Design review of the part built by this model. Coordinates are the model's own, in mm. Give positions to 0.01 mm unless a question says otherwise; leave off trailing zeros. Loops run counter-clockwise (first coordinate to the right, second up) from the corner with the lowest first, then second, coordinate; pieces in that order, holes last. Notation, with made-up numbers: (24, 28.5) - (66, 28.5) arc R14 cw to (66, 45.5) - close; hole circle Ø1 at (85.25, 58). An arc over 180 degrees is marked (long way). One line per item, written item: value. Start each with the question number.
```python
from build123d import *

# Parameters (mm, degrees)
SKETCH1_R           = 37.5
SKETCH1_R_2         = 26
SKETCH1_R_3         = 1
SKETCH1_R_4         = 1.5
BOSS_EXTRUDE1_DEPTH = 7


with BuildPart() as part:
    # Sketch1 → Boss-Extrude1 (new body)
    with BuildSketch(Plane(origin=(0, 0, 0), x_dir=(1, 0, 0), z_dir=(0, 1, 0))):
        with Locations(Location((0, 0, 0), (0, 0, 270))):
            Circle(SKETCH1_R)
        with Locations(Location((0, 0, 0), (0, 0, 270))):
            Circle(SKETCH1_R_2, mode=Mode.SUBTRACT)
        with Locations(Location((0, 30, 0), (0, 0, 270))):
            Circle(SKETCH1_R_3, mode=Mode.SUBTRACT)
        with Locations(Location((25.980762114, 15, 0), (0, 0, 270))):
            Circle(SKETCH1_R_3, mode=Mode.SUBTRACT)
        with Locations(Location((25.980762114, -15, 0), (0, 0, 270))):
            Circle(SKETCH1_R_3, mode=Mode.SUBTRACT)
        with Locations(Location((0, -30, 0), (0, 0, 270))):
            Circle(SKETCH1_R_3, mode=Mode.SUBTRACT)
        with Locations(Location((-25.980762114, -15, 0), (0, 0, 270))):
            Circle(SKETCH1_R_3, mode=Mode.SUBTRACT)
        with Locations(Location((-25.980762114, 15, 0), (0, 0, 270))):
            Circle(SKETCH1_R_3, mode=Mode.SUBTRACT)
        with Locations(Location((-33.80740392, -9.058666579, 0), (0, 0, 270))):
            Circle(SKETCH1_R_4, mode=Mode.SUBTRACT)
        with Locations(Location((-33.80740392, 9.058666579, 0), (0, 0, 270))):
            Circle(SKETCH1_R_4, mode=Mode.SUBTRACT)
        with Locations(Location((-24.748737342, 24.748737342, 0), (0, 0, 270))):
            Circle(SKETCH1_R_4, mode=Mode.SUBTRACT)
        with Locations(Location((-9.058666579, 33.80740392, 0), (0, 0, 270))):
            Circle(SKETCH1_R_4, mode=Mode.SUBTRACT)
        with Locations(Location((9.058666579, 33.80740392, 0), (0, 0, 270))):
            Circle(SKETCH1_R_4, mode=Mode.SUBTRACT)
        with Locations(Location((24.748737342, 24.748737342, 0), (0, 0, 270))):
            Circle(SKETCH1_R_4, mode=Mode.SUBTRACT)
        with Locations(Location((33.80740392, 9.058666579, 0), (0, 0, 270))):
            Circle(SKETCH1_R_4, mode=Mode.SUBTRACT)
        with Locations(Location((33.80740392, -9.058666579, 0), (0, 0, 270))):
            Circle(SKETCH1_R_4, mode=Mode.SUBTRACT)
        with Locations(Location((24.748737342, -24.748737342, 0), (0, 0, 270))):
            Circle(SKETCH1_R_4, mode=Mode.SUBTRACT)
        with Locations(Location((9.058666579, -33.80740392, 0), (0, 0, 270))):
            Circle(SKETCH1_R_4, mode=Mode.SUBTRACT)
        with Locations(Location((-9.058666579, -33.80740392, 0), (0, 0, 270))):
            Circle(SKETCH1_R_4, mode=Mode.SUBTRACT)
        with Locations(Location((-24.748737342, -24.748737342, 0), (0, 0, 270))):
            Circle(SKETCH1_R_4, mode=Mode.SUBTRACT)
    extrude(amount=BOSS_EXTRUDE1_DEPTH)


solid = part.part
```
(1) Take a section at D-D on y = 2.5. State how many separate pieces and enclosed holes the cut face has, and give its area (3 significant figures).
(2) Take a section at A-A on z = -30. State the section outline as (x, y) points, and give its area (3 significant figures).
(3) Take a section at B-B on x = -21.5. State the section outline as (y, z) points, and give its area (3 significant figures).
(4) Draft analysis for pull direction Z (two halves, no side actions). For faces 1 (the flat face through (-22.05, 7, -14.06)), 2 (the cylindrical face through (-22.818, 3.451, -29.759)), 3 (the cylindrical face through (0, 3, -29)), state which applies: pulls with the +Z half, pulls with the -Z half, needs draft (parallel to the pull), parting line crosses it, or undercut.
(5) Take a section at C-C on x = 0. State the section outline as (y, z) points, and give its area (3 significant figures).
(6) For pin 1 Ø2 at (x, y) = (-21, 5.5) entering from -Z; pin 2 Ø3 at (y, z) = (1, -8.5) entering from +X; pin 3 Ø1 at (x, y) = (27, 4.5) entering from +Z, all flat-tipped, find the tip position at first contact; note any pin that passes through.
(7) To check wall thickness, follow L1, parallel to Z at x = -24, y = 4.75; L2, parallel to X at y = 5, z = -8; L3, parallel to X at y = 1.5, z = 15. State the ranges of each line that lie inside material, in increasing order. Write a range as from..to.
Here are the results:
1. separate pieces: 1
1. enclosed holes: 19
1. area: 2,190 mm²
2. outline: (-22.5, 0) - (-1, 0) - (-1, 7) - (-22.5, 7) - close; (1, 0) - (22.5, 0) - (22.5, 7) - (1, 7) - close
2. area: 301 mm²
3. outline: (0, -30.72) - (7, -30.72) - (7, -14.62) - (0, -14.62) - close; (0, 14.62) - (7, 14.62) - (7, 30.72) - (0, 30.72) - close
3. area: 225 mm²
4. face 1: needs draft
4. face 2: parting line crosses it
4. face 3: undercut
5. outline: (0, -37.5) - (7, -37.5) - (7, -31) - (0, -31) - close; (0, -29) - (7, -29) - (7, -26) - (0, -26) - close; (0, 26) - (7, 26) - (7, 29) - (0, 29) - close; (0, 31) - (7, 31) - (7, 37.5) - (0, 37.5) - close
5. area: 133 mm²
6. pin 1: z = -31.72
6. pin 2: x = 36.84
6. pin 3: z = 26.53
7. L1: -28.81..-26.05, -23.45..-10, 10..23.45, 26.05..28.81
7. L2: -36.64..-34.87, -32.74..-24.74, 24.74..32.74, 34.87..36.64
7. L3: -34.37..-26.98, -24.98..-21.24, 21.24..24.98, 26.98..34.37
